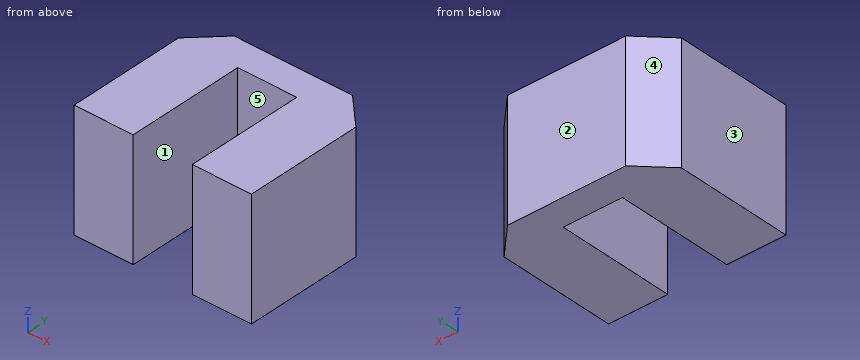
Autodesk Inventor part; units mm, degrees
ref_plane "YZ Plane" through (0, 0, 0) normal (1, 0, 0) x (0, 1, 0)
ref_plane "XZ Plane" through (0, 0, 0) normal (0, 1, 0) x (-1, 0, 0)
ref_plane "XY Plane" through (0, 0, 0) normal (0, 0, 1) x (1, 0, 0)
sketch "Sketch1" plane through (0, 0, 0) normal (0, 0, 1) x (1, 0, 0)
  line L0 (-4.7625, -6.35) -> (-1.5875, -6.35)
  line L1 (-1.5875, -6.35) -> (-1.5875, 0)
  line L2 (-1.5875, 0) -> (1.5875, 0)
  line L3 (1.5875, 0) -> (1.5875, -6.35)
  line L4 (1.5875, -6.35) -> (4.7625, -6.35)
  line L5 (4.7625, -6.35) -> (4.7625, 1.5875)
  line L6 (4.7625, 1.5875) -> (-4.7625, 1.5875)
  line L7 (-4.7625, 1.5875) -> (-4.7625, -6.35)
  point P0 (0, 0)
  point P1 (0, 0)
  point P2 (0, 1.5875)
  dimension "d0" = 3.175
  dimension "d1" = 3.175
  dimension "d2" = 6.35
  dimension "d3" = 1.5875
extrude "Extrusion1" add sketch "Sketch1" along normal blind 6.35
chamfer "Chamfer1" distance 1.5875 angle 45 2 edges at (-4.7625, 1.5875, 3.175) (4.7625, 1.5875, 3.175)
properties part number "3DPRINT,WIRE-GUARD,LOOP"
Geometry check sheet. Reference: the model listing, model coordinates, mm. Face numbers are marked on the shaded views. A direction names the side the tool comes from. Give positions to 0.01 mm unless a question says otherwise; leave off trailing zeros. Write each loop counter-clockwise with the first axis right and the second up, starting at its lowest first coordinate (ties: lowest second). Pieces come first, ordered by that corner, then holes.
1) Set-up check for the marked faces 4 and 5: record each of +Z, -Z, +X, -X, +Y, -Y from which the full face is reachable in a straight line by a thin tool's end or side.
Values follow:
face 4: +Z, -Z, -X, +Y
face 5: +Z, -Z, -Y
2) Cross-section at D-D (y = 0.5). Record the boundary of the cut face in (x, z).
Values follow:
outline: (-4.26, 0) - (4.26, 0) - (4.26, 6.35) - (-4.26, 6.35) - close
3) Cross-section at A-A (y = -0.5). Record the boundary of the cut face in (x, z).
Values follow:
outline: (-4.76, 0) - (-1.59, 0) - (-1.59, 6.35) - (-4.76, 6.35) - close; (1.59, 0) - (4.76, 0) - (4.76, 6.35) - (1.59, 6.35) - close
4) Release check for a two-part mould opening along X. For the marked faces 1, 2 and 3 record: released by +X, released by -X, zero draft, split by the parting line, or undercut.
Values follow:
face 1: undercut
face 2: zero draft
face 3: released by -X
5) Cross-section at C-C (x = 0.5). Record the boundary of the cut face in (y, z), plus the area to 3 significant figures.
Values follow:
outline: (0, 0) - (1.59, 0) - (1.59, 6.35) - (0, 6.35) - close
area: 10.1 mm2
6) Thickness scan on line 1 (X direction, y = -3.25, z = 5.5); line 2 (Y direction, x = 0, z = 1.75); line 3 (X direction, y = 1, z = 1). Record the ranges inside material, lowest first.
Values follow:
line 1: x = -4.76 to -1.59, 1.59 to 4.76
line 2: y = 0 to 1.59
line 3: x = -3.76 to 3.76
